Build history of the part. All positions in model axes, mm. Give positions to 0.01 mm unless a question says otherwise; leave off trailing zeros. Order: outer loops, then holes, each group sorted by start corner. A loop starts at its lowest first (then second) coordinate and runs counter-clockwise, first axis right, second up. Notation, with made-up numbers: M 16,62 L 33,62 A6 ccw 33,72 Z; hole C 29.5,2 d8. An arc over 180 degrees is marked long. One line per item, written item: value.
from build123d import *

# Parameters (mm, degrees)
F0_R     = 3.5
F0_R_2   = 1.5
F1_DEPTH = 2
F0_W     = 22.5
F0_H     = 32
F2_DEPTH = 4


with BuildPart() as f1:
    # F0 (on Top) → F1 (new body)
    with BuildSketch(Plane.XY):
        with BuildLine():
            ThreePointArc((20, 26.114874), (18.904278, 28.704066), (16.409269, 30))
            Line((16.409269, 30), (-16.409269, 30))
            ThreePointArc((-16.409269, 30), (-18.904278, 28.704066), (-20, 26.114874))
            Line((-20, 26.114874), (-20, 24.938533))
            ThreePointArc((-20, 24.938533), (-19.396294, 22.556811), (-17.73096, 20.750233))
            Line((-17.73096, 20.750233), (-13, 17.665434))
            Line((-13, 17.665434), (-13, 18))
            Line((-13, 18), (13, 18))
            Line((13, 18), (13, 17.665434))
            Line((13, 17.665434), (17.73096, 20.750233))
            ThreePointArc((17.73096, 20.750233), (19.396294, 22.556811), (20, 24.938533))
            Line((20, 24.938533), (20, 26.114874))
        make_face()
        with Locations((-15, 25)):
            Circle(F0_R, mode=Mode.SUBTRACT)
        Polygon((-9.18, 27), (-9.18, 28), (-8.18, 28), (8.18, 28), (9.170838, 28), (9.170838, 27), (9.170838, 21), (9.170838, 20), (8.18, 20), (-8.18, 20), (-9.18, 20), (-9.18, 21), align=None, mode=Mode.SUBTRACT)
        with Locations((15, 25)):
            Circle(F0_R, mode=Mode.SUBTRACT)
        with BuildLine():
            Line((17.73096, -20.750233), (13, -17.665434))
            Line((13, -17.665434), (13, -18))
            Line((13, -18), (-13, -18))
            Line((-13, -18), (-13, -17.665434))
            Line((-13, -17.665434), (-17.73096, -20.750233))
            ThreePointArc((-17.73096, -20.750233), (-19.396294, -22.556811), (-20, -24.938533))
            Line((-20, -24.938533), (-20, -26.114874))
            ThreePointArc((-20, -26.114874), (-18.904278, -28.704066), (-16.409269, -30))
            Line((-16.409269, -30), (16.409269, -30))
            ThreePointArc((16.409269, -30), (18.904278, -28.704066), (20, -26.114874))
            Line((20, -26.114874), (20, -24.938533))
            ThreePointArc((20, -24.938533), (19.396294, -22.556811), (17.73096, -20.750233))
        make_face()
        with Locations((-15, -25)):
            Circle(F0_R, mode=Mode.SUBTRACT)
        Polygon((-8.18, -20), (8.18, -20), (9.170838, -20), (9.170838, -21), (9.170838, -27), (9.170838, -28), (8.18, -28), (-8.18, -28), (-9.18, -28), (-9.18, -27), (-9.18, -21), (-9.18, -20), align=None, mode=Mode.SUBTRACT)
        with Locations((15, -25)):
            Circle(F0_R, mode=Mode.SUBTRACT)
        with Locations((-15, -25)):
            Circle(F0_R)
        with Locations((-15, -25)):
            Circle(F0_R_2, mode=Mode.SUBTRACT)
        with Locations((15, -25)):
            Circle(F0_R)
        with Locations((15, -25)):
            Circle(F0_R_2, mode=Mode.SUBTRACT)
        with Locations((15, 25)):
            Circle(F0_R)
        with Locations((15, 25)):
            Circle(F0_R_2, mode=Mode.SUBTRACT)
        with Locations((-15, 25)):
            Circle(F0_R)
        with Locations((-15, 25)):
            Circle(F0_R_2, mode=Mode.SUBTRACT)
        Polygon((-8.18, 28), (-9.18, 28), (-9.18, 27), (-1.743927, 24), (-9.18, 21), (-9.18, 20), (-8.18, 20), (0, 23.300129), (8.18, 20), (9.170838, 20), (9.170838, 21), (1.734764, 24), (9.170838, 27), (9.170838, 28), (8.18, 28), (0, 24.699871), align=None)
        Polygon((9.170838, -20), (8.18, -20), (0, -23.300129), (-8.18, -20), (-9.18, -20), (-9.18, -21), (-1.743927, -24), (-9.18, -27), (-9.18, -28), (-8.18, -28), (0, -24.699871), (8.18, -28), (9.170838, -28), (9.170838, -27), (1.734764, -24), (9.170838, -21), align=None)
    extrude(amount=F1_DEPTH)

    # F0 (on Top) → F2 (join)
    with BuildSketch(Plane.XY):
        Polygon((13, -17.665434), (13, 17.665434), (13, 18), (-13, 18), (-13, 17.665434), (-13, -17.665434), (-13, -18), (13, -18), align=None)
        Rectangle(F0_W, F0_H, mode=Mode.SUBTRACT)
    extrude(amount=F2_DEPTH)


solid = f1.part
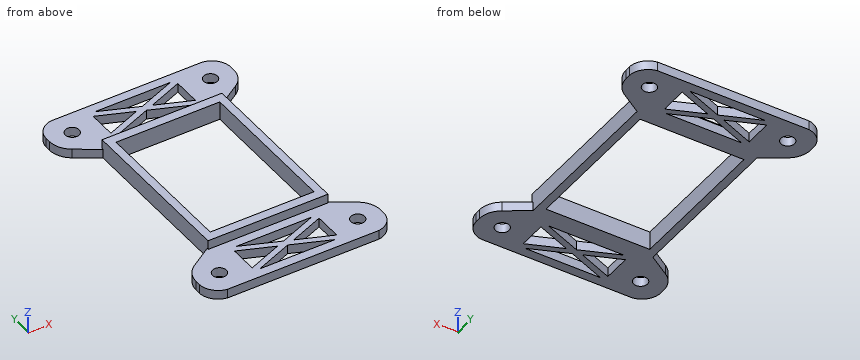
1) Pin check, flat tips, straight feed: pin 1 (1.6 mm diameter, centred on x = -2, z = 3, fed in from +Y); pin 2 (1.5 mm diameter, centred on y = 4, z = 1.5, fed in from +X); pin 3 (4 mm diameter, centred on x = -15, y = 25, fed in from -Z); pin 4 (0.6 mm diameter, centred on x = -3, z = 3, fed in from -Y). Stop position of each tip, or through.
Check values:
pin 1: y = 18
pin 2: x = 13
pin 3: z = 0
pin 4: y = -18
2) Saw through at C-C, the plane x = -15. Write the cut outline in (y, z), then the cut area to 3 significant figures.
Check values:
outline: M -30,0 L -26.5,0 L -26.5,2 L -30,2 Z; M -23.5,0 L -18.97,0 L -18.97,2 L -23.5,2 Z; M 18.97,0 L 23.5,0 L 23.5,2 L 18.97,2 Z; M 26.5,0 L 30,0 L 30,2 L 26.5,2 Z
area: 32.1 mm^2
3) Saw through at D-D, the plane x = -7. Give the number of separate pieces and of enclosed holes in the cut face, then the cut area to 3 significant figures.
Check values:
separate pieces: 8
enclosed holes: 0
area: 43.2 mm^2
4) Saw through at A-A, the plane y = 4.5. Write the cut outline in (x, z).
Check values:
outline: M -13,0 L -11.25,0 L -11.25,4 L -13,4 Z; M 11.25,0 L 13,0 L 13,4 L 11.25,4 Z
5) Drill centre lines: probe 1 along Y at (x, z) = (10.5, 2.75); probe 2 along Y at (x, z) = (-15, 0.6); probe 3 along X at (y, z) = (-3, 2.9). Where is each one in solid material? Low to high. Write a range as from..to.
Check values:
probe 1: -18..-16, 16..18
probe 2: -30..-26.5, -23.5..-18.97, 18.97..23.5, 26.5..30
probe 3: -13..-11.25, 11.25..13
6) Saw through at B-B, the plane z = 3.15. Write the cut outline in (x, y).
Check values:
outline: M -13,-18 L 13,-18 L 13,18 L -13,18 Z; hole M -11.25,-16 L 11.25,-16 L 11.25,16 L -11.25,16 Z
